Drawing for the job (mm, zero at the part's lowest x, y, z). A direction names the side the tool comes from. Give positions to 0.01 mm unless a question says otherwise; leave off trailing zeros. Loops run counter-clockwise (first coordinate to the right, second up) from the corner with the lowest first, then second, coordinate; pieces in that order, holes last.
1) Band-saw the part on C-C on z = 1.4. List the corners of the cut face in (x, y), then the cut area to 3 significant figures.
2) Band-saw the part on D-D on x = 20. List the corners of the cut face in (y, z), then the cut area to 3 significant figures.
3) Flat gauge pins, fed straight in: P1, Ø0.9, axis at y = 9, z = 1.5, coming from the -X side; P2, Ø1.5, axis at y = 9.5, z = 3, coming from the +X side; P3, Ø3, axis at x = 4, y = 53, coming from the +Z side. Where does each tip first touch, or does it go through?
4) Band-saw the part on A-A on y = 4. List the corners of the cut face in (x, z), then the cut area to 3 significant figures.
5) Wall check: line 1 (Y direction, x = 4, z = 3.05); line 2 (Y direction, x = 44, z = 0.35); line 3 (Y direction, x = 57.5, z = 3.2). Give the ranges that are in metal, low to high.
6) Two-plate mould, pull along Y, no slides. Class the marked faces 1, 2 and 3: +Y half, -Y half, draft (parallel to the pull), parting line (faces both ways), or undercut.
7) Band-saw the part on B-B on x = 56. List the corners of the cut face in (y, z).
8) 3-axis set-ups, long thin cutter, end or side, ignore diameter. For the marked faces 4, 5 and 6: which of +Z, -Z, +X, -X, +Y, -Y reach the whole face in a straight line?
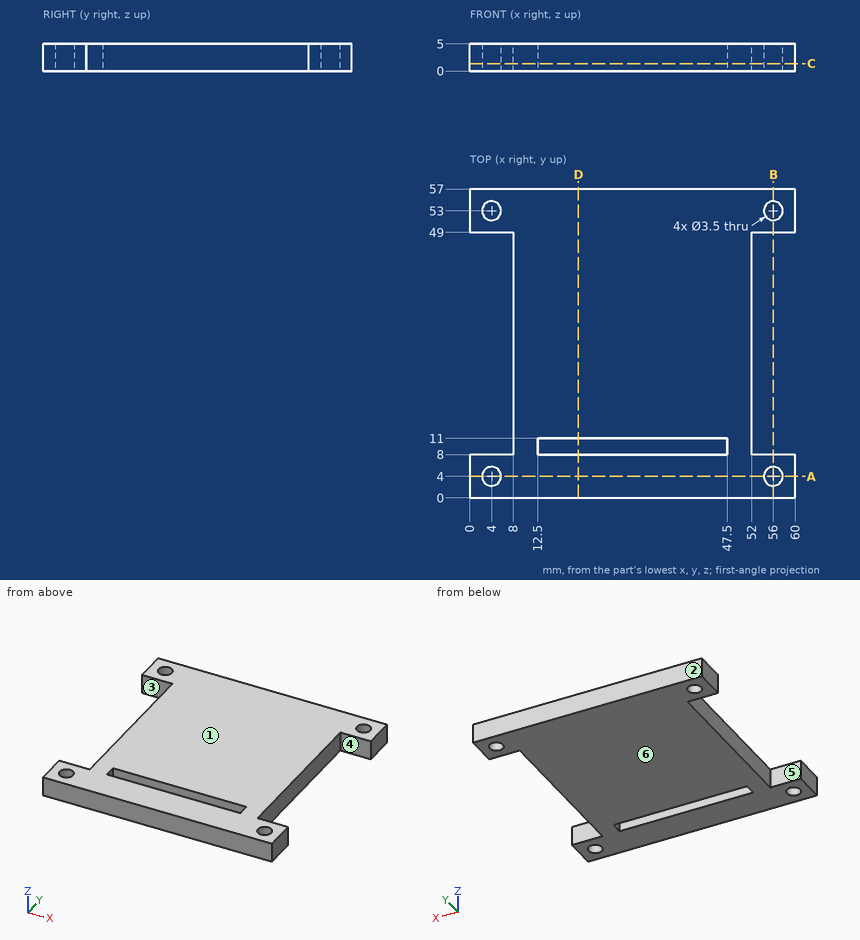
Findings below:
1. outline: (0, 0) - (60, 0) - (60, 8) - (52, 8) - (52, 49) - (60, 49) - (60, 57) - (0, 57) - (0, 49) - (8, 49) - (8, 8) - (0, 8) - close; hole circle Ø3.5 at (4, 4); hole circle Ø3.5 at (4, 53); hole (12.5, 8) - (47.5, 8) - (47.5, 11) - (12.5, 11) - close; hole circle Ø3.5 at (56, 4); hole circle Ø3.5 at (56, 53)
1. area: 2,620 mm2
2. outline: (0, 0) - (8, 0) - (8, 5) - (0, 5) - close; (11, 0) - (57, 0) - (57, 5) - (11, 5) - close
2. area: 270 mm2
3. P1: stops at x = 8
3. P2: stops at x = 52
3. P3: passes through
4. outline: (0, 0) - (2.25, 0) - (2.25, 5) - (0, 5) - close; (5.75, 0) - (54.25, 0) - (54.25, 5) - (5.75, 5) - close; (57.75, 0) - (60, 0) - (60, 5) - (57.75, 5) - close
4. area: 265 mm2
5. line 1: y = 0 to 2.25, 5.75 to 8, 49 to 51.25, 54.75 to 57
5. line 2: y = 0 to 8, 11 to 57
5. line 3: y = 0 to 3.1, 4.9 to 8, 49 to 52.1, 53.9 to 57
6. face 1: draft
6. face 2: +Y half
6. face 3: undercut
7. outline: (0, 0) - (2.25, 0) - (2.25, 5) - (0, 5) - close; (5.75, 0) - (8, 0) - (8, 5) - (5.75, 5) - close; (49, 0) - (51.25, 0) - (51.25, 5) - (49, 5) - close; (54.75, 0) - (57, 0) - (57, 5) - (54.75, 5) - close
8. face 4: +Z, -Z, +X
8. face 5: +Z, -Z, -X
8. face 6: -Z, +X, -X, +Y, -Y
